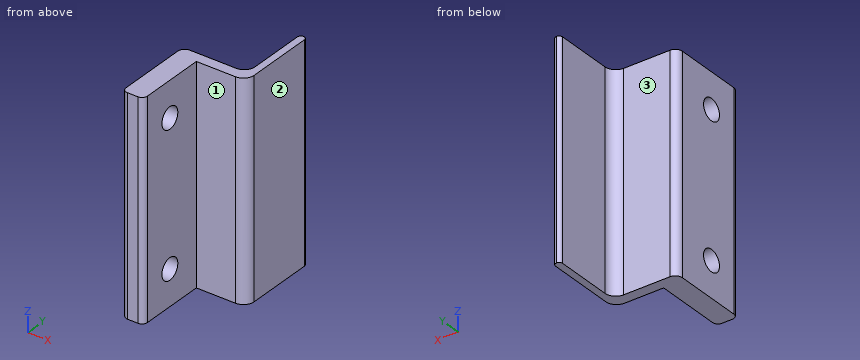
Autodesk Inventor part; units mm, degrees
ref_plane "YZ Plane" through (0, 0, 0) normal (1, 0, 0) x (0, 1, 0)
ref_plane "XZ Plane" through (0, 0, 0) normal (0, 1, 0) x (-1, 0, 0)
ref_plane "XY Plane" through (0, 0, 0) normal (0, 0, 1) x (1, 0, 0)
sketch "Sketch1" plane through (0, 0, 0) normal (0, 1, 0) x (-1, 0, 0)
  line L0 (0, 0) -> (20, 0)
  line L1 (20, 0) -> (20, -60)
  line L2 (20, -60) -> (0, -60)
  line L3 (0, -60) -> (0, 0)
  dimension "d0" = 20
  dimension "d1" = 60
extrude "Extrusion1" add sketch "Sketch1" along normal blind 3
sketch "Sketch2" plane through (0, 3, 0) normal (0, 1, 0) x (1, 0, 0)
  line L0 (-20, 0) -> (0, 0)
  line L1 (0, 0) -> (-2, 0)
  line L2 (-2, 0) -> (-2, 60)
  line L3 (-2, 60) -> (0, 60)
  line L4 (0, 60) -> (0, 0)
  dimension "d4" = 2
  dimension "d5" = 60
extrude "Extrusion2" add sketch "Sketch2" along normal blind 20
sketch "Sketch3" plane through (0, 0, 0) normal (0, -1, 0) x (1, 0, 0)
  line L0 (-20, 0) -> (0, 0)
  line L1 (0, -60) -> (-20, -60)
  line L2 (-20, 0) -> (-14, 0)
  line L3 (-14, 0) -> (-14, -60)
  line L4 (-14, -60) -> (-20, -60)
  line L5 (-20, -60) -> (-20, 0)
  point P0 (-14, 0)
  dimension "d8" = 6
extrude "Extrusion3" add sketch "Sketch3" along normal blind 20
sketch "Sketch4" plane through (-14, 0, 0) normal (1, 0, 0) x (0, 0, -1)
  line L0 (0, -20) -> (0, 0)
  line L1 (0, -10) -> (10, -10)
  line L2 (60, 0) -> (60, -20)
  circle A0 centre (10, -10) radius 3
  line L3 (60, -20) -> (0, -20)
  line L4 (0, -20) -> (60, -20)
  circle A1 centre (50, -10) radius 3
  point P0 (0, 3)
  point P1 (-60, -3)
  dimension "d11" = 10
  dimension "d12" = 6
  dimension "d15" = 40
extrude "Extrusion4" cut sketch "Sketch4" against normal through all
fillet "Fillet3" radius 3 2 edges at (-2, 3, -30) (0, 0, -30)
fillet "Fillet4" radius 1 2 edges at (0, 23, -30) (-2, 23, -30)
fillet "Fillet6" radius 1.5 2 edges at (-20, -20, -30) (-14, -20, -30)
fillet "Fillet10" radius 2 1 edges at (-20, 3, -30)
properties part number "CableChain_Holder"
Here's how the part is built. I have some questions about the finished solid (model axes, mm). Face numbers are marked on the shaded views. A direction names the side the tool comes from. Round coordinates to 2 decimals unless told otherwise and drop trailing zeros. Loops run counter-clockwise (first coordinate to the right, second up) from the corner with the lowest first, then second, coordinate; pieces in that order, holes last. Notation, with made-up numbers: (-28, 72.5) -> (27, 72.5) arc R19 cw to (27, 107.5) -> close; hole circle Ø8 at (6, 57). An arc over 180 degrees is marked (long way). Answer as CSV lines item,"result". Start each with the question number.
1. Imagine slicing it at A-A on y = -10. Write out the boundary of the cut face in (x, z), plus the area to 3 significant figures.
2. I need wall thicknesses on probe 1 along Y at (x, z) = (-18.25, -10); probe 2 along Y at (x, z) = (-13, -5.5); probe 3 along X at (y, z) = (-8.5, -57). Which ranges of each line are inside material? Lowest first, please. Write a range as from..to.
3. Imagine slicing it at D-D on y = 20. Write out the boundary of the cut face in (x, z).
4. For the marked faces 1, 2 and 3, which set-ups out of +Z, -Z, +X, -X, +Y, -Y let a thin tool reach every point of the face, with its end or its side?
5. I'm going to push flat-ended pins straight in: P1, Ø3, axis at x = -16.5, z = -17.5, coming from the +Y side; P2, Ø5, axis at y = 11.5, z = -15.5, coming from the -X side; P3, Ø15, axis at y = -13, z = -44.5, coming from the +X side. Where does each tip first touch, or does it pass through?
Solution:
1,outline,"(-20, -60) -> (-14, -60) -> (-14, -53) -> (-20, -53) -> close; (-20, -47) -> (-14, -47) -> (-14, -13) -> (-20, -13) -> close; (-20, -7) -> (-14, -7) -> (-14, 0) -> (-20, 0) -> close"
1,area,"288 mm²"
2,probe 1,"-20..-13, -7..2.98"
2,probe 2,"0..3"
2,probe 3,"-20..-14"
3,outline,"(-2, -60) -> (0, -60) -> (0, 0) -> (-2, 0) -> close"
4,face 1,"+Z, -Z, +X, -Y"
4,face 2,"+Z, -Z, +X, +Y, -Y"
4,face 3,"+Z, -Z, -X, +Y"
5,P1,"y = 3"
5,P2,"x = -2"
5,P3,"x = -14"
